Can you work these out from the model? Positions are in its coordinate system, mm. Coordinates: 2 decimals unless noted, no trailing zeros. Order: outer loops, then holes, each group sorted by start corner. A loop starts at its lowest first (then second) coordinate and runs counter-clockwise, first axis right, second up. Notation, with made-up numbers: (44, 56) -> (53, 56) arc R23 cw to (53, 85) -> close; hole circle Ø4 at (-30.75, 70). An arc over 180 degrees is marked (long way). Use a Markdown table: item, result. Add a question column.
1. Suppose I cut it at B-B, the plane x = -28.25. List the corners of the cut face in (y, z) for me.
2. Suppose I cut it at A-A, the plane z = 6. List the corners of the cut face in (x, y) for me, then the cut area to 3 significant figures.
3. For pin 1 Ø4 at (y, z) = (5, 9.5) entering from +X; pin 2 Ø1 at (y, z) = (24.5, 10) entering from +X; pin 3 Ø6 at (x, z) = (-21.5, 12.5) entering from -Y, each with a flat end and sliding along its axis, tell me the tip position at first contact or that it passes through.
4. Suppose I cut it at C-C, the plane y = 13. List the corners of the cut face in (x, z) for me, then the cut area to 3 significant figures.
5. If I drill on line 1 along Y through (x, z) = (-19.25, 12.5); line 2 along X through (y, z) = (1, 12.5); line 3 along X through (y, z) = (27, 3), over which ranges is the centre line in solid material (lowest first)? Write a range as from..to.
```python
from build123d import *

# Parameters (mm, degrees)
F1_DEPTH = 15


with BuildPart() as f1:
    # F0 (on Top) → F1 (new body)
    with BuildSketch(Plane.XY):
        with BuildLine():
            ThreePointArc((-24.649322, 26.966004), (-19.199356, 29.079291), (-16.921483, 34.462543))
            ThreePointArc((-16.921483, 34.462543), (-16.923414, 34.632717), (-16.929205, 34.802804))
            ThreePointArc((-16.929205, 34.802804), (-19.158107, 39.80547), (-24.193644, 41.959081))
            Line((-24.193644, 41.959081), (-24.421483, 34.462543))
            Line((-24.421483, 34.462543), (-24.649322, 26.966004))
        make_face()
        with BuildLine():
            ThreePointArc((-16.929205, 34.802804), (-16.923414, 34.632717), (-16.921483, 34.462543))
            ThreePointArc((-16.921483, 34.462543), (-19.199356, 29.079291), (-24.649322, 26.966004))
            Line((-24.649322, 26.966004), (-24.960474, 16.728221))
            ThreePointArc((-24.960474, 16.728221), (-18.298251, 13.907425), (-15.282183, 7.3313))
            Line((-15.282183, 7.3313), (-16.929205, 34.802804))
        make_face()
        with BuildLine():
            Line((-24.960474, 16.728221), (-24.649322, 26.966004))
            ThreePointArc((-24.649322, 26.966004), (-30.074188, 29.533352), (-31.879268, 35.257174))
            Line((-31.879268, 35.257174), (-35.191567, 7.936397))
            ThreePointArc((-35.191567, 7.936397), (-31.781704, 14.317222), (-24.960474, 16.728221))
        make_face()
        with BuildLine():
            ThreePointArc((-31.879268, 35.257174), (-30.074188, 29.533352), (-24.649322, 26.966004))
            Line((-24.649322, 26.966004), (-24.421483, 34.462543))
            Line((-24.421483, 34.462543), (-24.193644, 41.959081))
            ThreePointArc((-24.193644, 41.959081), (-29.350673, 40.115248), (-31.879268, 35.257174))
        make_face()
        with BuildLine():
            ThreePointArc((-15.264259, 6.732836), (-15.268741, 7.032202), (-15.282183, 7.3313))
            ThreePointArc((-15.282183, 7.3313), (-18.298251, 13.907425), (-24.960474, 16.728221))
            Line((-24.960474, 16.728221), (-25.264259, 6.732836))
            Line((-25.264259, 6.732836), (-25.568044, -3.262549))
            ThreePointArc((-25.568044, -3.262549), (-18.301424, -0.444833), (-15.264259, 6.732836))
        make_face()
        with BuildLine():
            Line((-25.264259, 6.732836), (-24.960474, 16.728221))
            ThreePointArc((-24.960474, 16.728221), (-31.781704, 14.317222), (-35.191567, 7.936397))
            ThreePointArc((-35.191567, 7.936397), (-32.848645, 0.215391), (-25.568044, -3.262549))
            Line((-25.568044, -3.262549), (-25.264259, 6.732836))
        make_face()
    extrude(amount=F1_DEPTH)


solid = f1.part
```
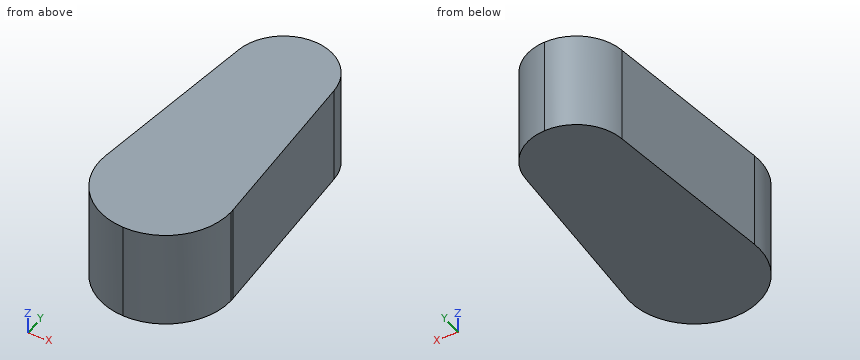
Worked out:
| question | item | result |
|---|---|---|
| 1 | outline | (-2.81, 0) -> (40.91, 0) -> (40.91, 15) -> (-2.81, 15) -> close |
| 2 | outline | (-35.19, 7.94) arc R10 ccw (long way) to (-15.26, 6.73) arc R10 ccw to (-15.28, 7.33) -> (-16.93, 34.8) arc R7.5 ccw to (-24.19, 41.96) arc R7.5 ccw to (-31.88, 35.26) -> close |
| 2 | area | 733 mm² |
| 3 | pin 1 | stops at x = -15.26 |
| 3 | pin 2 | stops at x = -16.28 |
| 3 | pin 3 | stops at y = -3.24 |
| 4 | outline | (-34.58, 0) -> (-15.62, 0) -> (-15.62, 15) -> (-34.58, 15) -> close |
| 4 | area | 284 mm² |
| 5 | line 1 | y = -1.26..39.89 |
| 5 | line 2 | x = -33.46..-17.07 |
| 5 | line 3 | x = -32.88..-16.46 |
